Autodesk Fusion 360 part; units mm, degrees
sketch "Sketch1" plane through (0, 0, 0) normal (0, 1, 0) x (1, 0, 0)
  line L0 (-50, 50) -> (50, 50)
  line L1 (50, 50) -> (50, -20)
  line L2 (50, -20) -> (-25, -20)
  line L3 (-50, 0) -> (-50, 50)
  line L4 (-25, -20) -> (-50, 0)
extrude "Extrude1" add sketch "Sketch1" along normal blind 20
sketch "Sketch2" plane through (0, 20, 0) normal (0, 1, 0) x (-1, 0, 0)
  line L0 (25, 20) -> (-50, 20)
  line L1 (-50, 20) -> (-50, -50)
  line L2 (-50, -50) -> (50, -50)
  line L3 (50, -50) -> (50, 0)
  line L4 (50, 0) -> (25, 20)
  line L5 (-50, 20) -> (-50, -50)
  line L6 (25, 20) -> (-50, 20)
  line L7 (50, 0) -> (25, 20)
  line L8 (50, -50) -> (50, 0)
  line L9 (-50, -50) -> (50, -50)
  line L10 (50, -40) -> (26.5041, -40)
  line L11 (26.5041, -40) -> (-1.6201, -17.5006)
  line L12 (-1.6201, -17.5006) -> (-30, -17.5006)
  line L13 (-30, -17.5006) -> (-30, 5.9595)
  line L14 (-30, 5.9595) -> (-40, 20)
  circle A0 centre (-13.6491, -35.3724) radius 5.4442
  line L15 (-30, -17.5006) -> (-30, -50)
extrude "Extrude2" add sketch "Sketch2" along normal blind 15 contours L2 L3 L8 L9 L10 L11 L12 L15
extrude "Extrude3" add sketch "Sketch2" along normal blind 30 contours L0 L1 L2 L5 L6 L9 L13 L14 L15
sketch "Sketch3" plane through (30, 0, 0) normal (-1, 0, 0) x (0, 0, 1)
  line L0 (-50, 35) -> (-17.5006, 35)
  line L1 (-17.5006, 35) -> (-17.5006, 20)
  line L2 (-17.5006, 20) -> (5.9595, 20)
  line L3 (5.9595, 20) -> (5.9595, 50)
  line L4 (5.9595, 50) -> (-50, 50)
  line L5 (-50, 50) -> (-50, 35)
  circle A0 centre (-5, 30) radius 4.5807
extrude "Extrude4" cut sketch "Sketch3" along normal through all contours A0
The model under review builds one solid part; all positions refer to its coordinate system, in mm. A direction names the side the tool comes from. Round coordinates to 2 decimals unless told otherwise and drop trailing zeros. Loops run counter-clockwise (first coordinate to the right, second up) from the corner with the lowest first, then second, coordinate; pieces in that order, holes last. Notation, with made-up numbers: (-40, 8) - (-30, 8) arc R37 cw to (-30, 46) - close; hole circle Ø2 at (41.25, 56). An arc over 180 degrees is marked (long way). Use a Markdown table: item, result. Add a question column.
Q1. Add section B-B (x = 28.5). State the section outline as (y, z) points.
Q2. For probe 1 along X at (y, z) = (45, -19); probe 2 along X at (y, z) = (8, 8); probe 3 along Y at (x, z) = (14.5, -5), list the stretches that pass through material, from the lowest coordinate up.
Q3. The part is to be moulded in two halves that separate along Z. For faces 4 (the face through (17.662, 27.395, -39.052)), 5 (the face through (-1, 35, -37)), 6 (the face through (-12.64, 27.4, -28.91)), say which applies: pulls with the +Z half, pulls with the -Z half, needs draft (parallel to the pull), parting line crosses it, or undercut.
Q4. Add section A-A (y = 3.5). State the section outline as (x, z) points.
Q5. Machinability: for faces 1 (the face through (14, 20, -35)), 2 (the face through (12, 14, 20)), 3 (the face through (34.93, 34.79, 12.88)), which of the approach directions +Z, -Z, +X, -X, +Y, -Y give a long, thin tool a straight path to every point of the face, cutting with its end or side? Answer none if there is none.
Q6. Add section C-C (z = -7). State the section outline as (x, y) points, plus the area to 3 significant figures.
Q7. Add section D-D (y = 28). State the section outline as (x, z) points.
Q8. Insertion check: pin 1 Ø1.5 at (x, y) = (-29.5, 12.5) entering from +Z; pin 2 Ø4.5 at (x, y) = (12.5, 27) entering from +Z; pin 3 Ø10 at (x, z) = (13.65, -35.37) entering from +Y. Each pin has a flat end and moves straight along its axis. Give the tip position at first contact, or say it passes through.
Worked answers:
| question | item | result |
|---|---|---|
| 1 | outline | (0, -50) - (35, -50) - (35, -17.5) - (20, -17.5) - (20, 20) - (0, 20) - close |
| 2 | probe 1 | 30 to 50 |
| 2 | probe 2 | -40 to 50 |
| 2 | probe 3 | 0 to 20 |
| 3 | face 4 | undercut |
| 3 | face 5 | needs draft |
| 3 | face 6 | pulls with the +Z half |
| 4 | outline | (-50, -50) - (50, -50) - (50, 20) - (-25, 20) - (-50, 0) - close |
| 5 | face 1 | +Y |
| 5 | face 2 | +Z, +X, -X, +Y, -Y |
| 5 | face 3 | +Z, -X, +Y |
| 6 | outline | (-50, 0) - (50, 0) - (50, 50) - (30, 50) - (30, 20) - (-50, 20) - close |
| 6 | area | 2,600 mm² |
| 7 | outline | (-50, -50) - (50, -50) - (50, 20) - (40, 20) - (30, 5.96) - (30, -17.5) - (1.62, -17.5) - (-26.5, -40) - (-50, -40) - close; hole circle Ø10.89 at (13.65, -35.37) |
| 8 | pin 1 | z = 17 |
| 8 | pin 2 | z = -17.5 |
| 8 | pin 3 | y = 20 |
